Can you work these out from the drawing? Everything is in mm from the part's minimum corner. Coordinates: 2 decimals unless noted, no trailing zeros. Loops run counter-clockwise (first coordinate to the right, second up) from the corner with the lowest first, then second, coordinate; pieces in that order, holes last.
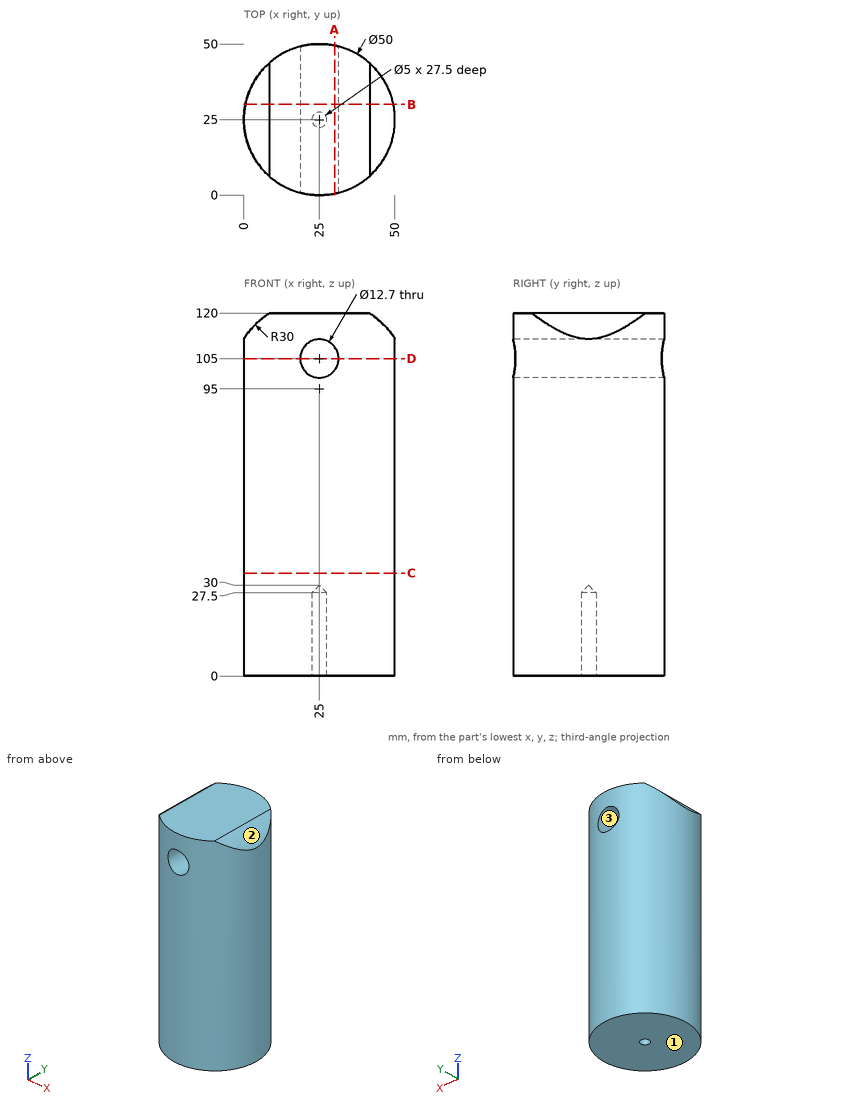
1) We'd pull the mould along Z, two halves only. Please class the marked faces 1, 2 and 3: released by +Z, released by -Z, zero draft, split by the parting line, or undercut.
2) If I drill on L1, parallel to Z at x = 25, y = 31.5; L2, parallel to Y at x = 25, z = 18; L3, parallel to Z at x = 19.5, y = 8.5, over which ranges is the centre line in solid material (lowest first)?
3) Will these pins go through, and if not, where does the flat tip stop? pin 1 (8 mm diameter, centred on x = 44, z = 20, fed in from -Y); pin 2 (3 mm diameter, centred on x = 38.5, z = 22.5, fed in from +Y); pin 3 (10 mm diameter, centred on y = 34.5, z = 69.5, fed in from -X).
4) Imagine slicing it at C-C on z = 34. List the corners of the cut face in (x, y) for me, plus the area to 3 significant figures.
5) Imagine slicing it at A-A on x = 30. List the corners of the cut face in (y, z) for me, plus the area to 3 significant figures.
6) Imagine slicing it at D-D on z = 105. List the corners of the cut face in (x, y) for me, plus the area to 3 significant figures.
7) Imagine slicing it at B-B on y = 30. List the corners of the cut face in (x, z) for me, plus the area to 3 significant figures.
Solved:
1. face 1: released by -Z
1. face 2: released by +Z
1. face 3: undercut
2. L1: z = 0 to 98.65, 111.35 to 120
2. L2: y = 0 to 22.5, 27.5 to 50
2. L3: z = 0 to 101.83, 108.17 to 120
3. pin 1: stops at y = 5
3. pin 2: stops at y = 46.93
3. pin 3: stops at x = 0.41
4. outline: circle Ø50 at (25, 25)
4. area: 1,960 mm2
5. outline: (0.51, 0) - (49.49, 0) - (49.49, 101.09) - (0.51, 101.09) - close; (0.51, 108.91) - (49.49, 108.91) - (49.49, 120) - (0.51, 120) - close
5. area: 5,500 mm2
6. outline: (18.65, 0.82) - (18.65, 49.18) arc R25 ccw to start; (31.35, 0.82) arc R25 ccw to (31.35, 49.18) - close
6. area: 1,340 mm2
7. outline: (0.51, 0) - (49.49, 0) - (49.49, 112.32) arc R30 ccw to (41.58, 120) - (8.42, 120) arc R30 ccw to (0.51, 112.32) - close; hole circle Ø12.7 at (25, 105)
7. area: 5,700 mm2
